Build history of the part. All positions in model axes, mm. A direction names the side the tool comes from. Round coordinates to 2 decimals unless told otherwise and drop trailing zeros. Write each loop counter-clockwise with the first axis right and the second up, starting at its lowest first coordinate (ties: lowest second). Pieces come first, ordered by that corner, then holes.
Item 1: Band-saw the part on A-A, the plane x = 0. Write the cut outline in (y, z), then the cut area to 3 significant figures.
Item 2: Band-saw the part on D-D, the plane y = 42. Write the cut outline in (x, z), then the cut area to 3 significant figures.
Item 3: Drop flat-ended pins along their axis: pin 1 Ø4 at (y, z) = (30, 3.5) entering from -X; pin 2 Ø1.5 at (x, z) = (4, 5.5) entering from +Y; pin 3 Ø2 at (x, z) = (8.5, 3) entering from -Y. Give the stop position or say it passes through.
Item 4: Mould opens along Y. For faces 1 (the flat face through (9.803, 54.071, 4.93)), 2 (the flat face through (14.47, 34, 5)), 3 (the flat face through (2.303, 13.198, 4.93)), 4 (the cylindrical face through (-1.5, 0.07, 4.93)) say: +Y half, -Y half, draft (parallel to the pull), parting line (faces both ways), or undercut.
Item 5: Wall check: probe 1 along Y at (x, z) = (0, 3); probe 2 along X at (y, z) = (44, 6.5); probe 3 along Y at (x, z) = (2.75, 6) (3 decimals). Give the ranges that are in metal, low to high.
Item 6: 3-axis set-ups, long thin cutter, end or side, ignore diameter. For faces 5 (the flat face through (8, 34, 5)), 6 (the flat face through (8, 23, 0)): which of +Z, -Z, +X, -X, +Y, -Y reach the whole face in a straight line?
Item 7: Band-saw the part on C-C, the plane y = 0. Write the cut outline in (x, z).
```python
from build123d import *

# Parameters (mm, degrees)
SKETCH_1_R      = 1.5
EXTRUDE_1_DEPTH = 10


with BuildPart() as part:
    # 草图1 → 凸台-拉伸1 (new body)
    with BuildSketch(Plane.XY):
        with BuildLine():
            Line((8, 44.424510324), (8, 24.249761918))
            Line((8, 24.249761918), (-3.555429037, 1.832736851))
            ThreePointArc((-3.555429037, 1.832736851), (-1.832736851, -3.555429037), (3.555429037, -1.832736851))
            Line((3.555429037, -1.832736851), (3.554621026, -1.832320341))
            Line((3.554621026, -1.832320341), (3.593691894, -1.756524572))
            Line((3.593691894, -1.756524572), (14.47, 19.343035702))
            Line((14.47, 19.343035702), (14.47, 48.303035702))
            Line((14.47, 48.303035702), (5.002811382, 60.002387807))
            Line((5.002811382, 60.002387807), (8, 44.424510324))
        make_face()
        Circle(SKETCH_1_R, mode=Mode.SUBTRACT)
    extrude(amount=EXTRUDE_1_DEPTH)


solid = part.part
```
Results:
1. outline: (-4, 0) - (-1.5, 0) - (-1.5, 10) - (-4, 10) - close; (1.5, 0) - (8.73, 0) - (8.73, 10) - (1.5, 10) - close
1. area: 97.3 mm2
2. outline: (8, 0) - (14.47, 0) - (14.47, 10) - (8, 10) - close
2. area: 64.7 mm2
3. pin 1: stops at x = 8
3. pin 2: stops at y = 17.94
3. pin 3: stops at y = 5.82
4. face 1: +Y half
4. face 2: draft
4. face 3: undercut
4. face 4: undercut
5. probe 1: y = -4 to -1.5, 1.5 to 8.73
5. probe 2: x = 8 to 14.47
5. probe 3: y = -2.905 to 14.065
6. face 5: +Z, -Z, -X
6. face 6: -Z, +X, -X, +Y, -Y
7. outline: (-4, 0) - (-1.5, 0) - (-1.5, 10) - (-4, 10) - close; (1.5, 0) - (4.5, 0) - (4.5, 10) - (1.5, 10) - close
